Source: three-view drawing plus pictorial views. Frame: mm from the lowest corner of the part. A direction names the side the tool comes from. Give positions to 0.01 mm unless a question says otherwise; leave off trailing zeros. Write each loop counter-clockwise with the first axis right and the second up, starting at its lowest first coordinate (ties: lowest second). Pieces come first, ordered by that corner, then holes. Notation, with made-up numbers: (79.25, 85) -> (111.25, 85) arc R27 cw to (111.25, 101) -> close; hole circle Ø7 at (52.25, 37.5). An arc over 180 degrees is marked (long way). Answer in a Markdown table with one row per item. Add a question column.
Item 1: Section query C-C on x = 49.5. Output: boundary loops of the cut face in (y, z), plus the area to 3 significant figures.
Item 2: Material intervals for probe 1 along Z at (x, y) = (29.5, 24.75); probe 2 along Y at (x, z) = (29.5, 1.5); probe 3 along Z at (x, y) = (20.5, 43.5), sorted ascending. Write a range as from..to.
Item 3: Section query A-A on y = 29.5. Output: boundary loops of the cut face in (x, z), plus the area to 3 significant figures.
Item 4: Draft query along Y for the marked faces 1, 2 and 3. Return one class per face: +Y half, -Y half, draft (parallel to the pull), parting line (faces both ways), or undercut.
Item 5: First-contact query: P1, Ø7, axis at x = 50.07, y = 41.38, coming from the -Z side; P2, Ø3, axis at x = 29.5, z = 10, coming from the +Y side; P3, Ø6, axis at x = 40.5, y = 39.5, coming from the +Z side; P4, Ø4.5, axis at x = 29.5, z = 10, coming from the +Y side. Flat tips, straight axial feed; report the tip coordinate or a pass-through.
Item 6: Section query B-B on x = 29.5. Output: boundary loops of the cut face in (y, z), plus the area to 3 significant figures.
Item 7: Section query D-D on z = 11. Output: boundary loops of the cut face in (x, y), plus the area to 3 significant figures.
Item 8: Access query for the marked faces 4 and 5. Directions: +Z, -Z, +X, -X, +Y, -Y. A direction counts if a zero-diameter tool reaches every point of the face in a straight line with its end or side. Return the directions, or none.
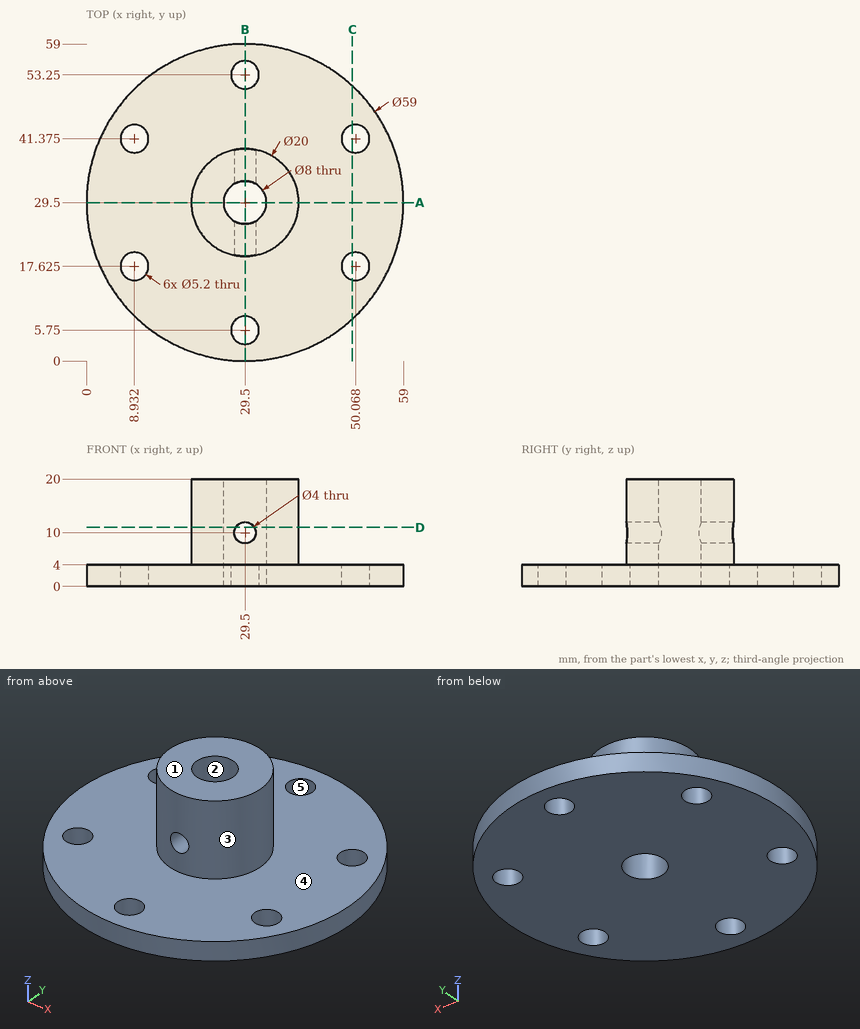
Findings below:
| question | item | result |
|---|---|---|
| 1 | outline | (7.81, 0) -> (15.09, 0) -> (15.09, 4) -> (7.81, 4) -> close; (20.16, 0) -> (38.84, 0) -> (38.84, 4) -> (20.16, 4) -> close; (43.91, 0) -> (51.19, 0) -> (51.19, 4) -> (43.91, 4) -> close |
| 1 | area | 133 mm^2 |
| 2 | probe 1 | z = 0..8, 12..20 |
| 2 | probe 2 | y = 0..3.15, 8.35..25.5, 33.5..50.65, 55.85..59 |
| 2 | probe 3 | z = 0..4 |
| 3 | outline | (0, 0) -> (25.5, 0) -> (25.5, 20) -> (19.5, 20) -> (19.5, 4) -> (0, 4) -> close; (33.5, 0) -> (59, 0) -> (59, 4) -> (39.5, 4) -> (39.5, 20) -> (33.5, 20) -> close |
| 3 | area | 396 mm^2 |
| 4 | face 1 | draft |
| 4 | face 2 | undercut |
| 4 | face 3 | parting line |
| 5 | P1 | stops at z = 0 |
| 5 | P2 | passes through |
| 5 | P3 | stops at z = 4 |
| 5 | P4 | stops at y = 39.5 |
| 6 | outline | (0, 0) -> (3.15, 0) -> (3.15, 4) -> (0, 4) -> close; (8.35, 0) -> (25.5, 0) -> (25.5, 8) -> (19.5, 8) -> (19.5, 4) -> (8.35, 4) -> close; (19.5, 12) -> (25.5, 12) -> (25.5, 20) -> (19.5, 20) -> close; (33.5, 0) -> (50.65, 0) -> (50.65, 4) -> (39.5, 4) -> (39.5, 8) -> (33.5, 8) -> close; (33.5, 12) -> (39.5, 12) -> (39.5, 20) -> (33.5, 20) -> close; (55.85, 0) -> (59, 0) -> (59, 4) -> (55.85, 4) -> close |
| 6 | area | 306 mm^2 |
| 7 | outline | (27.77, 19.65) -> (27.77, 25.89) arc R4 cw to (27.77, 33.11) -> (27.77, 39.35) arc R10 ccw to start; (31.23, 19.65) arc R10 ccw to (31.23, 39.35) -> (31.23, 33.11) arc R4 cw to (31.23, 25.89) -> close |
| 7 | area | 222 mm^2 |
| 8 | face 4 | +Z |
| 8 | face 5 | +Z, -Z |
